CAD build for the part. Positions are in the model's coordinates, mm. Face numbers are marked on the shaded views. A direction names the side the tool comes from. Round coordinates to 2 decimals unless told otherwise and drop trailing zeros. Order: outer loops, then holes, each group sorted by start corner. A loop starts at its lowest first (then second) coordinate and runs counter-clockwise, first axis right, second up. Notation, with made-up numbers: M -18,-12.5 L -6,-12.5 A11 cw -6,6.5 Z; hole C 36.25,-33.75 d10. An arc over 180 degrees is marked long. Answer as a JSON object with one key per item and string values.
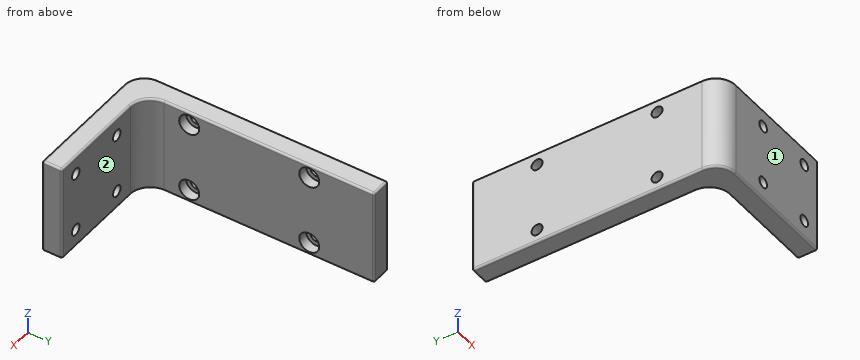
```python
from build123d import *

# Parameters (mm, degrees)
BASE_DEPTH                           = 48
ROOT_EDGE_FILLET_R                   = 10
SLIDER_BOLT_HOLE_PATTERN_D           = 5.5
SLIDER_BOLT_HOLE_PATTERN_CBORE_D     = 10
SLIDER_BOLT_HOLE_PATTERN_CBORE_DEPTH = 5
DESKTOP_BOLT_HOLE_PATTERN_D          = 5.5
EXTERNAL_FILLET_R                    = 1


with BuildPart() as part:
    # Sketch1 → base (new body)
    with BuildSketch(Plane.XY):
        Polygon((0, 125), (0, 0), (70, 0), (70, 10), (10, 10), (10, 125), align=None)
    extrude(amount=BASE_DEPTH)

    # root_edge_fillet
    root_edge_fillet_edges = [part.edges().sort_by_distance(p)[0] for p in [
        (10, 10, 24),
        (0, 0, 24),
    ]]
    fillet(root_edge_fillet_edges, radius=ROOT_EDGE_FILLET_R)

    # slider_bolt_hole_pattern (through all)
    with Locations(Plane(origin=(10, 0, 0), x_dir=(0, 0, -1), z_dir=(1, 0, 0))):
        with Locations((-41.5, 92.5), (-6.5, 32.5), (-41.5, 32.5), (-6.5, 92.5)):
            CounterBoreHole(SLIDER_BOLT_HOLE_PATTERN_D / 2, SLIDER_BOLT_HOLE_PATTERN_CBORE_D / 2, SLIDER_BOLT_HOLE_PATTERN_CBORE_DEPTH)

    # desktop_bolt_hole_pattern (through all)
    with Locations(Plane(origin=(0, 10, 0), x_dir=(1, 0, 0), z_dir=(0, 1, 0))):
        with Locations((30, -9), (60, -39), (30, -39), (60, -9)):
            Hole(DESKTOP_BOLT_HOLE_PATTERN_D / 2)

    # external_fillet
    external_fillet_edges = [part.edges().sort_by_distance(p)[0] for p in [
        (10, 125, 24),
        (70, 10, 24),
        (70, 0, 24),
        (0, 125, 24),
        (70, 5, 48),
        (45, 10, 48),
        (40, 0, 0),
        (40, 0, 48),
        (10, 72.5, 0),
        (2.928932188, 2.928932188, 0),
        (10, 72.5, 48),
        (2.928932188, 2.928932188, 48),
        (12.928932188, 12.928932188, 0),
        (12.928932188, 12.928932188, 48),
        (5, 125, 48),
        (45, 10, 0),
        (70, 5, 0),
        (0, 67.5, 48),
        (0, 67.5, 0),
        (5, 125, 0),
    ]]
    fillet(external_fillet_edges, radius=EXTERNAL_FILLET_R)


solid = part.part
```
Item 1: Saw through at C-C on z = 43. List the corners of the cut face in (x, y).
Worked answers:
{"outline": "M 0,10 A10 ccw 10,0 L 69,0 A1 ccw 70,1 L 70,9 A1 ccw 69,10 L 20,10 A10 cw 10,20 L 10,27.73 L 5,27.73 L 5,30.2 L 0,30.2 Z; M 0,34.8 L 5,34.8 L 5,37.27 L 10,37.27 L 10,87.73 L 5,87.73 L 5,90.2 L 0,90.2 Z; M 0,94.8 L 5,94.8 L 5,97.27 L 10,97.27 L 10,124 A1 ccw 9,125 L 1,125 A1 ccw 0,124 Z"}
Item 2: Drop flat-ended pins along their axis: pin 1 Ø14 at (y, z) = (83.5, 31.5) entering from +X; pin 2 Ø8 at (y, z) = (92.5, 6.5) entering from +X; pin 3 Ø9 at (x, z) = (60, 39) entering from +Y. Give the stop position or say it passes through.
Worked answers:
{"pin 1": "stops at x = 10", "pin 2": "stops at x = 5", "pin 3": "stops at y = 10"}
Item 3: Saw through at B-B on x = 30. List the corners of the cut face in (y, z), and give its area (3 significant figures).
Worked answers:
{"outline": "M 0,1 A1 ccw 1,0 L 9,0 A1 ccw 10,1 L 10,6.25 L 0,6.25 Z; M 0,11.75 L 10,11.75 L 10,36.25 L 0,36.25 Z; M 0,41.75 L 10,41.75 L 10,47 A1 ccw 9,48 L 1,48 A1 ccw 0,47 Z", "area": "369 mm2"}
Item 4: Saw through at D-D on z = 32. List the corners of the cut face in (x, y), and give its area (3 significant figures).
Worked answers:
{"outline": "M 0,10 A10 ccw 10,0 L 69,0 A1 ccw 70,1 L 70,9 A1 ccw 69,10 L 20,10 A10 cw 10,20 L 10,124 A1 ccw 9,125 L 1,125 A1 ccw 0,124 Z", "area": "1,850 mm2"}
Item 5: 3-axis set-ups, long thin cutter, end or side, ignore diameter. For the marked faces 1 and 2: which of +Z, -Z, +X, -X, +Y, -Y reach the whole face in a straight line?
Worked answers:
{"face 1": "+Z, -Z, +X, -X, -Y", "face 2": "+Z, -Z, +X, +Y"}
Item 6: Saw through at A-A on y = 32.5. List the corners of the cut face in (x, z).
Worked answers:
{"outline": "M 0,1 A1 ccw 1,0 L 9,0 A1 ccw 10,1 L 10,1.5 L 5,1.5 L 5,3.75 L 0,3.75 Z; M 0,9.25 L 5,9.25 L 5,11.5 L 10,11.5 L 10,36.5 L 5,36.5 L 5,38.75 L 0,38.75 Z; M 0,44.25 L 5,44.25 L 5,46.5 L 10,46.5 L 10,47 A1 ccw 9,48 L 1,48 A1 ccw 0,47 Z"}
Item 7: Wall check: line 1 along Z through (x, y) = (6, 32); line 2 along Z through (x, y) = (30, 3.5); line 3 along Y through (x, z) = (3, 6.5). Give the ranges that are in metal, low to high. Write a range as [from, to].
Worked answers:
{"line 1": "z = [0, 1.53], [11.47, 36.53], [46.47, 48]", "line 2": "z = [0, 6.25], [11.75, 36.25], [41.75, 48]", "line 3": "y = [2.86, 29.75], [35.25, 89.75], [95.25, 125]"}
